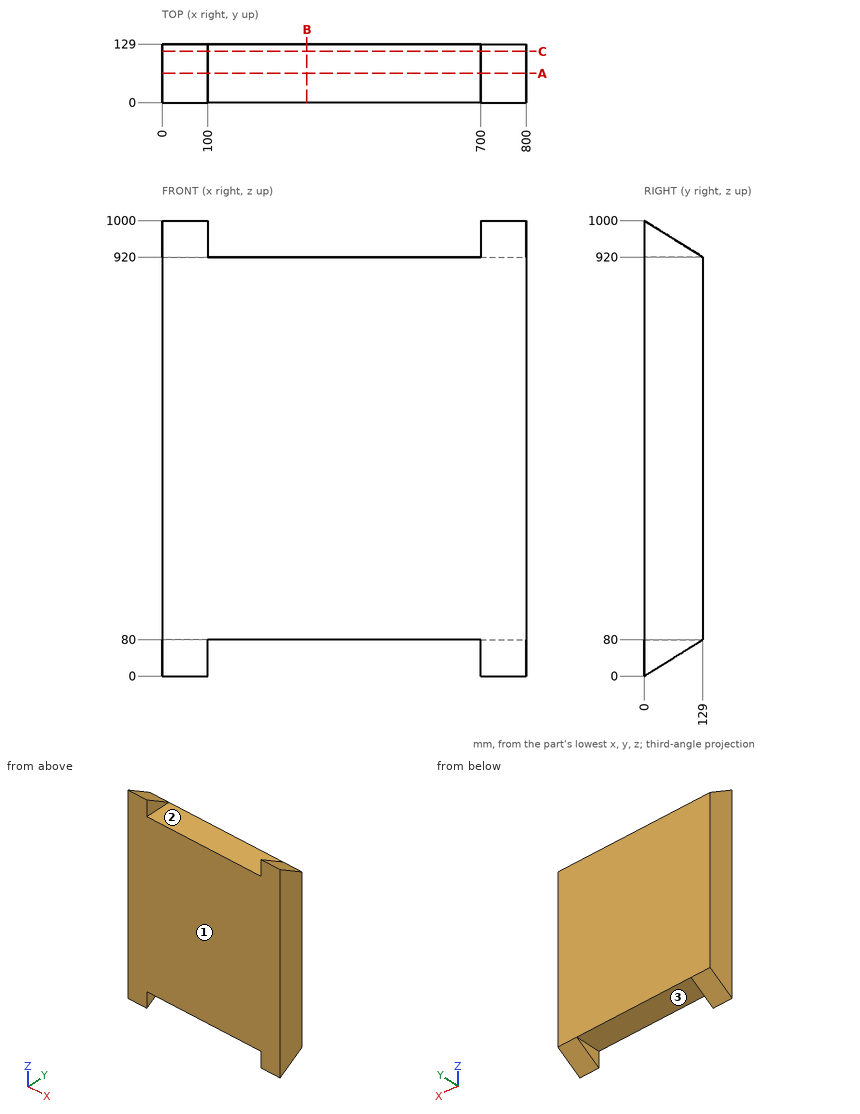
Geometry: see drawing. Coordinates: mm, zero at the bounding-box minimum. A direction names the side the tool comes from. Round coordinates to 2 decimals unless told otherwise and drop trailing zeros. Order: outer loops, then holes, each group sorted by start corner. A loop starts at its lowest first (then second) coordinate and runs counter-clockwise, first axis right, second up. Notation, with made-up numbers: (45, 28.25) - (56, 28.25) arc R22 cw to (56, 40.25) - close; hole circle Ø8 at (-7.5, -36.5). An arc over 180 degrees is marked (long way). Use a Markdown table: item, result. Add a question column.
1. Section query C-C (y = 113). Return the cut outline in (x, z), then the cut area to 3 significant figures.
2. Set-up query: the marked faces 1, 2 and 3. Return all of +Z, -Z, +X, -X, +Y, -Y with unobstructed straight access to the full face (end or side cutting, diameter ignored); none if empty.
3. Line query: probe 1 along X at (y, z) = (80, 938.5); probe 2 along Z at (x, y) = (525, 47); probe 3 along Y at (x, z) = (745.5, 75.5). Output: solid intervals per line, ascending.
4. Section query B-B (x = 318). Return the cut outline in (y, z), then the cut area to 3 significant figures.
5. Section query A-A (y = 64.5). Return the cut outline in (x, z), then the cut area to 3 significant figures.
6. First-contact query: pin 1 (10 mm diameter, centred on x = 319, y = 56, fed in from +Z); pin 2 (6 mm diameter, centred on x = 209.5, y = 57, fed in from -Z). Flat tips, straight axial feed; report the tip coordinate or a pass-through.
Derived:
| question | item | result |
|---|---|---|
| 1 | outline | (0, 70.08) - (100, 70.08) - (100, 80) - (700, 80) - (700, 70.08) - (800, 70.08) - (800, 929.92) - (700, 929.92) - (700, 920) - (100, 920) - (100, 929.92) - (0, 929.92) - close |
| 1 | area | 676,000 mm2 |
| 2 | face 1 | +Z, -Z, +X, -X, -Y |
| 2 | face 2 | +Z, +Y, -Y |
| 2 | face 3 | -Z, +Y, -Y |
| 3 | probe 1 | 0 to 100, 700 to 800 |
| 3 | probe 2 | 80 to 920 |
| 3 | probe 3 | 0 to 121.74 |
| 4 | outline | (0, 80) - (129, 80) - (129, 920) - (0, 920) - close |
| 4 | area | 108,000 mm2 |
| 5 | outline | (0, 40) - (100, 40) - (100, 80) - (700, 80) - (700, 40) - (800, 40) - (800, 960) - (700, 960) - (700, 920) - (100, 920) - (100, 960) - (0, 960) - close |
| 5 | area | 688,000 mm2 |
| 6 | pin 1 | z = 920 |
| 6 | pin 2 | z = 80 |
